from build123d import *

# Parameters (mm, degrees)
BOSS_EXTRUDE1_DEPTH     = 4.2
SKETCH3_R               = 5
BOSS_EXTRUDE2_DEPTH     = 0.5
CUT_EXTRUDE1_REACH      = 11.7
SKETCH4_R               = 2.5
CUT_EXTRUDE2_REACH      = 18.251
CUT_EXTRUDE2_END_RADIUS = 2.5
SKETCH5_R               = 1


with BuildPart() as part:
    # Sketch1 → Boss-Extrude1 (new body)
    with BuildSketch(Plane(origin=(0, 0, 0), x_dir=(1, 0, 0), z_dir=(0, 1, 0))):
        Polygon((-4, 6), (-6, 4), (-6, -4), (-4, -6), (4, -6), (6, -4), (6, 4), (4, 6), align=None)
    extrude(amount=BOSS_EXTRUDE1_DEPTH)

    # Sketch3 → Boss-Extrude2 (add)
    with BuildSketch(Plane(origin=(0, 4.2, 0), x_dir=(1, 0, 0), z_dir=(0, 1, 0))):
        with Locations(Location((0, 0, 0), (0, 0, 270))):
            Circle(SKETCH3_R)
    extrude(amount=BOSS_EXTRUDE2_DEPTH)

    # Sketch4 → Cut-Extrude1 (cut, up to next)
    with BuildSketch(Plane(origin=(0, 4.7, 0), x_dir=(1, 0, 0), z_dir=(0, 1, 0)), mode=Mode.PRIVATE) as cut_extrude1_sk1:
        with Locations(Location((0, 0, 0), (0, 0, 270))):
            Circle(SKETCH4_R)
    cut_extrude1_tool1 = extrude(cut_extrude1_sk1.sketch, amount=-CUT_EXTRUDE1_REACH, mode=Mode.PRIVATE) & part.part
    add(cut_extrude1_tool1.solids().sort_by_distance((0, 4.7, 0))[0], mode=Mode.SUBTRACT)

    # Cut-Extrude2: up to this cylinder (the profile starts outside it)
    cut_extrude2_end = Plane(origin=(0, 2.1, 0), z_dir=(0, 1, 0)) * Cylinder(CUT_EXTRUDE2_END_RADIUS, 42.502, mode=Mode.PRIVATE)
    # Sketch5 → Cut-Extrude2 (cut, up to the surface)
    with BuildSketch(Plane(origin=(5, 0, 5), x_dir=(0.7071067811865481, 0, -0.7071067811865469), z_dir=(0.7071067811865469, 0, 0.7071067811865481)), mode=Mode.PRIVATE) as cut_extrude2_sk1:
        with Locations((0, 2.1)):
            Circle(SKETCH5_R)
    cut_extrude2_tool1 = extrude(cut_extrude2_sk1.sketch, amount=-CUT_EXTRUDE2_REACH, mode=Mode.PRIVATE) - cut_extrude2_end
    add(cut_extrude2_tool1.solids().sort_by_distance((5, 2.1, 5))[0], mode=Mode.SUBTRACT)


solid = part.part
Model file for the job. Use its own axes, mm. A direction names the side the tool comes from. Give positions to 0.01 mm unless a question says otherwise; leave off trailing zeros. Loops run counter-clockwise (first coordinate to the right, second up) from the corner with the lowest first, then second, coordinate; pieces in that order, holes last. Notation, with made-up numbers: (-30.75, -10) -> (0.25, -10) arc R11 ccw to (0.25, 5) -> close; hole circle Ø5 at (89, -40). An arc over 180 degrees is marked (long way). Use a Markdown table: item, result. Add a question column.
(1) Slice it at C-C on y = 3.3. List the corners of the cut face in (x, z).
(2) Tool access for faces 1 (the cylindrical face through (-4.88, 4.45, -1.08)), 2 (the flat face through (-5, 2, -5)): list every direction of +Z, -Z, +X, -X, +Y, -Y with a clear straight run to the whole face (end or side of a thin tool).
(3) Mould opens along Z. For faces 3 (the cylindrical face through (-2.44, 2.38, -0.54)), 4 (the flat face through (-6, 2, 0)), 5 (the flat face through (-5, 2, 5)) say: +Z half, -Z half, draft (parallel to the pull), parting line (faces both ways), or undercut.
(4) Drop a flat-ended pin along its axis: pin 1 Ø3 at (x, z) = (-4.5, -2.5) entering from -Y. Give the stop position or say it passes through.
(5) Slice it at B-B on z = 0. List the corners of the cut face in (x, y).
(6) Wall check: line 1 along X through (y, z) = (3.7, 0); line 2 along Y through (x, z) = (3.25, -4.5); line 3 along Y through (x, z) = (2.5, 1.5). Give the ranges that are in metal, low to high.
(7) Slice it at D-D on x = -3.5. List the corners of the cut face in (y, z), and give its area (3 significant figures).
(8) Slice it at A-A on x = 0. List the corners of the cut face in (y, z), and give its area (3 significant figures).
Filled sheet:
| question | item | result |
|---|---|---|
| 1 | outline | (-6, -4) -> (-4, -6) -> (4, -6) -> (6, -4) -> (6, 4) -> (4, 6) -> (-4, 6) -> (-6, 4) -> close; hole circle Ø5 at (0, 0) |
| 2 | face 1 | +Y |
| 2 | face 2 | -Z, -X, +Y, -Y |
| 3 | face 3 | undercut |
| 3 | face 4 | draft |
| 3 | face 5 | +Z half |
| 4 | pin 1 | y = 0 |
| 5 | outline | (-6, 0) -> (-2.5, 0) -> (-2.5, 4.7) -> (-5, 4.7) -> (-5, 4.2) -> (-6, 4.2) -> close; (2.5, 0) -> (6, 0) -> (6, 4.2) -> (5, 4.2) -> (5, 4.7) -> (2.5, 4.7) -> close |
| 6 | line 1 | -6 to -2.5, 2.5 to 6 |
| 6 | line 2 | 0 to 4.2 |
| 6 | line 3 | 0 to 1.39, 2.81 to 4.7 |
| 7 | outline | (0, -6) -> (4.2, -6) -> (4.2, -3.57) -> (4.7, -3.57) -> (4.7, 3.57) -> (4.2, 3.57) -> (4.2, 6) -> (0, 6) -> close |
| 7 | area | 54.0 mm2 |
| 8 | outline | (0, -6) -> (4.2, -6) -> (4.2, -5) -> (4.7, -5) -> (4.7, -2.5) -> (0, -2.5) -> close; (0, 2.5) -> (4.7, 2.5) -> (4.7, 5) -> (4.2, 5) -> (4.2, 6) -> (0, 6) -> close |
| 8 | area | 31.9 mm2 |
